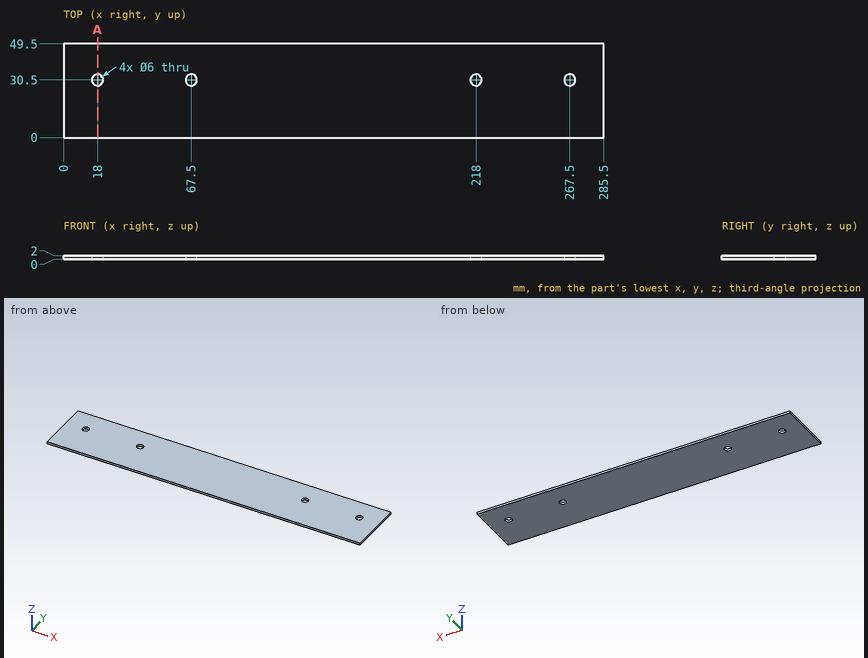
Job drawing, mm, ordinate dimensions from the low corner. One solid piece. Give positions to 0.01 mm unless a question says otherwise; leave off trailing zeros. Loops run counter-clockwise (first coordinate to the right, second up) from the corner with the lowest first, then second, coordinate; pieces in that order, holes last. Notation, with made-up numbers: (-36, 41.5) -> (-5, 41.5) arc R23 cw to (-5, 63.5) -> close; hole circle Ø10 at (-16.5, 88.5). An arc over 180 degrees is marked (long way). Write each question's results on one line, items separated by ' | '. Start each with the question number.
Q1. Pin check, flat tip, straight feed: P1, Ø5, axis at x = 18, y = 30.5, coming from the +Z side. Stop position of the tip, or through.
Q2. Band-saw the part on A-A on x = 18. List the corners of the cut face in (y, z), plus the area to 3 significant figures.
Q3. Wall check: L1, parallel to Y at x = 67.5, z = 0.8; L2, parallel to X at y = 28, z = 1.5; L3, parallel to Y at x = 70, z = 1.7. Give the ranges that are in metal, low to high.
Results are:
1) P1: passes through
2) outline: (0, 0) -> (27.5, 0) -> (27.5, 2) -> (0, 2) -> close; (33.5, 0) -> (49.5, 0) -> (49.5, 2) -> (33.5, 2) -> close | area: 87.0 mm²
3) L1: y = 0 to 27.5, 33.5 to 49.5 | L2: x = 0 to 16.34, 19.66 to 65.84, 69.16 to 216.34, 219.66 to 265.84, 269.16 to 285.5 | L3: y = 0 to 28.84, 32.16 to 49.5
